Here's how the part is built. I have some questions about the finished solid (model axes, mm). Give positions to 0.01 mm unless a question says otherwise; leave off trailing zeros. Loops run counter-clockwise (first coordinate to the right, second up) from the corner with the lowest first, then second, coordinate; pieces in that order, holes last.
Q1. Suppose I cut it at B-B (z = -6). List the corners of the cut face in (x, y) for me, and give its area (3 significant figures).
Q2. I need wall thicknesses on probe 1 along X at (y, z) = (-42, 0); probe 2 along Z at (x, y) = (77.6, -1.1) (3 decimals); probe 3 along Z at (x, y) = (-22, -17). Which ranges of each line are inside material? Lowest first, please.
Q3. Suppose I cut it at A-A (x = -29). List the corners of the cut face in (y, z) for me, and give its area (3 significant figures).
Q4. I'm going to push flat-ended pins straight in: P1, Ø0.8, axis at x = 85, y = -1, coming from the +Z side; P2, Ø6, axis at y = -11, z = 1, coming from the -X side; P3, Ø8, axis at y = -18.5, z = -11.5, coming from the +X side; P4, Ø12, axis at x = -13.5, z = -10, coming from the +Y side. Where does each tip first touch, or does it pass through?
Q5. Suppose I cut it at C-C (y = -12.5). List the corners of the cut face in (x, z) for me.
```python
from build123d import *

# Parameters (mm, degrees)
F1_DEPTH     = 50
F0_W         = 8
F0_H         = 8
F0_R         = 1.425
F2_DEPTH     = 1.6
F3_R         = 2
F5_R         = 2
F6_START     = 35
F0_W_2       = 4
F0_H_2       = 4
F0_R_2       = 0.9
F6_DEPTH     = 11
F7_T1_DEPTH  = 11
F7_T6_DEPTH  = 4
F7_S7_R      = 0.9
F7_T8_DEPTH  = 4
F7_T13_DEPTH = 9
F7_T17_DEPTH = 16
F7_T24_DEPTH = 9
F7_T28_DEPTH = 16
F7_T31_DEPTH = 21
F9_R         = 2


# Not quite as in the source:
# - a fillet or chamfer that OpenCascade refuses, or shapes differently, is made with other operations: its cross-section is extruded or revolved along the edge and cut away or added


with BuildPart() as f1:
    # F0 (on Front) → F1 (new body)
    with BuildSketch(Plane.XZ):
        Polygon((-81.6, -18.6015841149), (-81.6, -19.1), (-73.6, -19.1), (73.6, -19.1), (81.6, -19.1), (81.6, -18.6015841149), (81.6, -10.6015841149), (81.6, 10.6015841149), (81.6, 18.6015841149), (81.6, 19.1), (73.6, 19.1), (-73.6, 19.1), (-81.6, 19.1), (-81.6, 18.6015841149), (-81.6, 10.6015841149), (-81.6, -10.6015841149), align=None)
        Polygon((80, -2), (80, -17.5), (-80, -17.5), (-80, 17.5), (80, 17.5), (80, 2), align=None, mode=Mode.SUBTRACT)
    extrude(amount=F1_DEPTH)

    # F0 (on Front) → F2 (join)
    with BuildSketch(Plane.XZ):
        Polygon((-81.6, -18.6015841149), (-81.6, -19.1), (-73.6, -19.1), (73.6, -19.1), (81.6, -19.1), (81.6, -18.6015841149), (81.6, -10.6015841149), (81.6, 10.6015841149), (81.6, 18.6015841149), (81.6, 19.1), (73.6, 19.1), (-73.6, 19.1), (-81.6, 19.1), (-81.6, 18.6015841149), (-81.6, 10.6015841149), (-81.6, -10.6015841149), align=None)
        Polygon((80, -2), (80, -17.5), (-80, -17.5), (-80, 17.5), (80, 17.5), (80, 2), align=None, mode=Mode.SUBTRACT)
        with Locations((-77.6, -23.1)):
            Rectangle(F0_W, F0_H)
        with Locations((-77.6, -23.1)):
            Circle(F0_R, mode=Mode.SUBTRACT)
        with Locations((-85.6, -14.6015841149)):
            Rectangle(F0_W, F0_H)
        with Locations((-85.6, -14.6015841149)):
            Circle(F0_R, mode=Mode.SUBTRACT)
        with Locations((77.6, -23.1)):
            Rectangle(F0_W, F0_H)
        with Locations((77.6, -23.1)):
            Circle(F0_R, mode=Mode.SUBTRACT)
        with Locations((-85.6, 14.6015841149)):
            Rectangle(F0_W, F0_H)
        with Locations((-85.6, 14.6015841149)):
            Circle(F0_R, mode=Mode.SUBTRACT)
        with Locations((85.6, -14.6015841149)):
            Rectangle(F0_W, F0_H)
        with Locations((85.6, -14.6015841149)):
            Circle(F0_R, mode=Mode.SUBTRACT)
        with Locations((-77.6, 23.1)):
            Rectangle(F0_W, F0_H)
        with Locations((-77.6, 23.1)):
            Circle(F0_R, mode=Mode.SUBTRACT)
        with Locations((85.6, 14.6015841149)):
            Rectangle(F0_W, F0_H)
        with Locations((85.6, 14.6015841149)):
            Circle(F0_R, mode=Mode.SUBTRACT)
        with Locations((77.6, 23.1)):
            Rectangle(F0_W, F0_H)
        with Locations((77.6, 23.1)):
            Circle(F0_R, mode=Mode.SUBTRACT)
    extrude(amount=F2_DEPTH)

    # F3
    f3_edges = [f1.edges().sort_by_distance(p)[0] for p in [
        (-81.6, -0.8, 27.1),
        (-73.6, -0.8, 27.1),
        (73.6, -0.8, 27.1),
        (81.6, -0.8, 27.1),
        (89.6, -0.8, -10.601584),
        (89.6, -0.8, -18.601584),
        (81.6, -0.8, -27.1),
        (73.6, -0.8, -27.1),
        (-89.6, -0.8, -18.601584),
        (-89.6, -0.8, -10.601584),
        (-81.6, -0.8, -27.1),
    ]]
    fillet(f3_edges, radius=F3_R)

    # F4: F1 across plane


with BuildPart() as f1_1:
    add(f1.part)
    add(f1.part.mirror(Plane.YZ))

    # F5
    f5_edges = [f1_1.edges().sort_by_distance(p)[0] for p in [
        (-73.6, -0.8, -27.1),
        (73.6, -0.8, -27.1),
    ]]
    fillet(f5_edges, radius=F5_R)

    # F0 (on Front) → F6 (join)
    with BuildSketch(Plane.XZ.offset(F6_START)):
        with Locations((78, 0)):
            Rectangle(F0_W_2, F0_H_2)
        with Locations((78, 0)):
            Circle(F0_R_2, mode=Mode.SUBTRACT)
    extrude(amount=F6_DEPTH)

    # F7: fillet of radius 2 on 5 edges, made by hand

    # F7_s2 → F7_t1 (join)
    with BuildSketch(Plane.XZ.offset(35)):
        with BuildLine():
            ThreePointArc((80, -4), (79.4142135624, -2.5857864376), (78, -2))
            Line((78, -2), (80, -2))
            Line((80, -2), (80, -4))
        make_face()
        with BuildLine():
            ThreePointArc((80, 4), (79.4142135624, 2.5857864376), (78, 2))
            Line((78, 2), (80, 2))
            Line((80, 2), (80, 4))
        make_face()
    extrude(amount=F7_T1_DEPTH)


with BuildPart() as f7_tool4:
    # F7_s5 → F7_t6 (new body)
    with BuildSketch(Plane.XY.offset(-2)):
        with BuildLine():
            ThreePointArc((80, -33), (79.4142135624, -34.4142135624), (78, -35))
            Line((78, -35), (80, -35))
            Line((80, -35), (80, -33))
        make_face()
    extrude(amount=F7_T6_DEPTH)

    # F7_s7 → F7_t8 (cut, symmetric)
    with BuildSketch(Plane.XZ.offset(34)):
        with Locations((78, 0)):
            Circle(F7_S7_R)
    extrude(amount=F7_T8_DEPTH, both=True, mode=Mode.SUBTRACT)


with BuildPart() as f1_2:
    add(f1_1.part)

    # F7_t3: union F7_tool4
    add(f7_tool4.part)


with BuildPart() as f7_tool11:
    # F7_s12 → F7_t13 (new body)
    with BuildSketch(Plane.XY.offset(-7)):
        with BuildLine():
            ThreePointArc((80, -33), (79.4142135624, -34.4142135624), (78, -35))
            Line((78, -35), (80, -35))
            Line((80, -35), (80, -33))
        make_face()
    extrude(amount=F7_T13_DEPTH)

    split(bisect_by=Plane.XY.offset(-2), keep=Keep.BOTTOM)


with BuildPart() as f7_tool15:
    # F7_s16 → F7_t17 (new body)
    with BuildSketch(Plane.XZ.offset(30)):
        with BuildLine():
            ThreePointArc((80, -4), (79.4142135624, -2.5857864376), (78, -2))
            Line((78, -2), (80, -2))
            Line((80, -2), (80, -4))
        make_face()
    extrude(amount=F7_T17_DEPTH)

    split(bisect_by=Plane.XZ.offset(35), keep=Keep.BOTTOM)


with BuildPart() as f7_tool11_1:
    add(f7_tool11.part)

    # F7_t19: intersect F7_tool15
    add(f7_tool15.part, mode=Mode.INTERSECT)


with BuildPart() as f1_3:
    add(f1_2.part)

    # F7_t9: union F7_tool11
    add(f7_tool11_1.part)


with BuildPart() as f7_tool22:
    # F7_s23 → F7_t24 (new body)
    with BuildSketch(Plane.XY.offset(-2)):
        with BuildLine():
            ThreePointArc((80, -33), (79.4142135624, -34.4142135624), (78, -35))
            Line((78, -35), (80, -35))
            Line((80, -35), (80, -33))
        make_face()
    extrude(amount=F7_T24_DEPTH)

    split(bisect_by=Plane.XY.offset(2), keep=Keep.TOP)


with BuildPart() as f7_tool26:
    # F7_s27 → F7_t28 (new body)
    with BuildSketch(Plane.XZ.offset(30)):
        with BuildLine():
            ThreePointArc((80, 4), (79.4142135624, 2.5857864376), (78, 2))
            Line((78, 2), (80, 2))
            Line((80, 2), (80, 4))
        make_face()
    extrude(amount=F7_T28_DEPTH)

    split(bisect_by=Plane.XZ.offset(35), keep=Keep.BOTTOM)


with BuildPart() as f7_tool22_1:
    add(f7_tool22.part)

    # F7_t30: intersect F7_tool26
    add(f7_tool26.part, mode=Mode.INTERSECT)


with BuildPart() as f1_4:
    add(f1_3.part)

    # F7_t20: union F7_tool22
    add(f7_tool22_1.part)

    # F7_s32 → F7_t31 (cut)
    with BuildSketch(Plane.XZ.offset(30)):
        with BuildLine():
            ThreePointArc((78, -2), (76.5857864376, -1.4142135624), (76, 0))
            Line((76, 0), (76, -2))
            Line((76, -2), (78, -2))
        make_face()
        with BuildLine():
            ThreePointArc((78, 2), (76.5857864376, 1.4142135624), (76, 0))
            Line((76, 0), (76, 2))
            Line((76, 2), (78, 2))
        make_face()
    extrude(amount=F7_T31_DEPTH, mode=Mode.SUBTRACT)

    # F8: F1 across plane


with BuildPart() as f1_5:
    add(f1_4.part)
    add(f1_4.part.mirror(Plane.YZ))

    # F9
    f9_edges = [f1_5.edges().sort_by_distance(p)[0] for p in [
        (89.6, -0.8, 10.601584),
        (89.6, -0.8, 18.601584),
        (-89.6, -0.8, 10.601584),
        (-89.6, -0.8, 18.601584),
    ]]
    fillet(f9_edges, radius=F9_R)


solid = f1_5.part
```
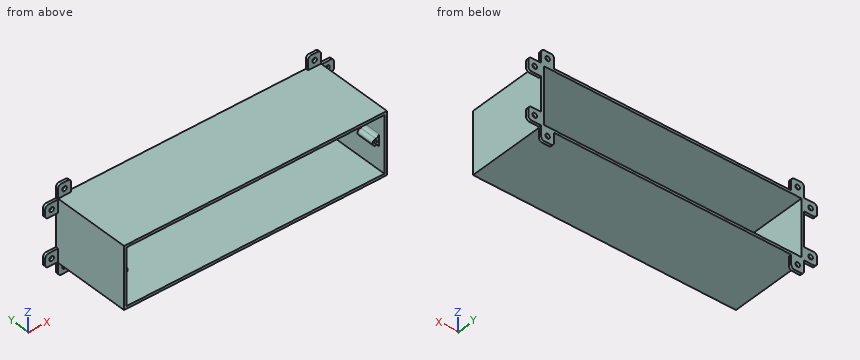
Solutions:
1. outline: (-81.6, -50) - (-80, -50) - (-80, 0) - (-81.6, 0) - close; (80, -50) - (81.6, -50) - (81.6, 0) - (80, 0) - close
1. area: 160 mm2
2. probe 1: x = -81.6 to -78.9, -77.1 to -76, 76 to 77.1, 78.9 to 81.6
2. probe 2: z = -27.1 to -24.525, -21.675 to -17.5, 17.5 to 21.675, 24.525 to 27.1
2. probe 3: z = -19.1 to -17.5, 17.5 to 19.1
3. outline: (-50, -19.1) - (0, -19.1) - (0, -17.5) - (-50, -17.5) - close; (-50, 17.5) - (0, 17.5) - (0, 19.1) - (-50, 19.1) - close
3. area: 160 mm2
4. P1: stops at z = 18.6
4. P2: stops at x = -81.6
4. P3: stops at x = 81.6
4. P4: passes through
5. outline: (-81.6, -19.1) - (81.6, -19.1) - (81.6, 19.1) - (-81.6, 19.1) - close; hole (-80, -17.5) - (80, -17.5) - (80, 17.5) - (-80, 17.5) - close
